```python
from build123d import *

# Parameters (mm, degrees)
SKETCH1_R           = 30
BOSS_EXTRUDE1_DEPTH = 2
SKETCH2_R           = 3.5
SKETCH2_R_2         = 2.5
BOSS_EXTRUDE2_DEPTH = 10
FILLET1_R           = 1
FILLET2_R           = 1


with BuildPart() as part:
    # Sketch1 → Boss-Extrude1 (new body)
    with BuildSketch(Plane(origin=(0, 0, 0), x_dir=(1, 0, 0), z_dir=(0, 1, 0))):
        with Locations(Location((0, 0, 0), (0, 0, 270))):
            Circle(SKETCH1_R)
    extrude(amount=BOSS_EXTRUDE1_DEPTH)

    # Sketch2 → Boss-Extrude2 (add)
    with BuildSketch(Plane.XZ):
        with Locations(Location((0, 0, 0), (0, 0, 90))):
            Circle(SKETCH2_R)
        with Locations(Location((0, 0, 0), (0, 0, 270))):
            Circle(SKETCH2_R_2, mode=Mode.SUBTRACT)
    extrude(amount=BOSS_EXTRUDE2_DEPTH)

    # Fillet1
    fillet1_edges = [part.edges().sort_by_distance(p)[0] for p in [
        (0, 0, -3.5),
    ]]
    fillet(fillet1_edges, radius=FILLET1_R)

    # Fillet2
    fillet2_edges = [part.edges().sort_by_distance(p)[0] for p in [
        (0, 0, 2.5),
    ]]
    fillet(fillet2_edges, radius=FILLET2_R)


solid = part.part
```
Geometry: final body of the model. Coordinates: model frame, mm. A direction names the side the tool comes from. Give positions to 0.01 mm unless a question says otherwise; leave off trailing zeros. Loops run counter-clockwise (first coordinate to the right, second up) from the corner with the lowest first, then second, coordinate; pieces in that order, holes last. Notation, with made-up numbers: (-12, -24.5) -> (20, -24.5) arc R30 ccw to (20, 2.5) -> close; hole circle Ø5 at (64, 51). An arc over 180 degrees is marked (long way). Return JSON: item names as keys, results as strings.
Item 1: Section A-A, the plane x = 0. Output: boundary loops of the cut face in (y, z).
Filled in:
{"outline": "(-10, -3.5) -> (-1, -3.5) arc R1 cw to (0, -4.5) -> (0, -30) -> (2, -30) -> (2, 30) -> (0, 30) -> (0, 4.5) arc R1 cw to (-1, 3.5) -> (-10, 3.5) -> (-10, 2.5) -> (-1, 2.5) arc R1 cw to (0, 1.5) -> (0, -1.5) arc R1 cw to (-1, -2.5) -> (-10, -2.5) -> close"}
Item 2: Pin query (flat end, axial travel): P1, Ø2, axis at x = 21, y = 0, coming from the +Z side; P2, Ø1.5, axis at y = -1, z = -7, coming from the -X side; P3, Ø8, axis at x = 0, z = 0, coming from the -Y side; P4, Ø3, axis at x = 1, z = 5.5, coming from the -Y side. Return the tip coordinate at first contact, or that it passes through.
Filled in:
{"P1": "z = 22.36", "P2": "through", "P3": "y = -10", "P4": "y = -0.09"}
Item 3: Section C-C, the plane y = -7.5. Output: boundary loops of the cut face in (x, z).
Filled in:
{"outline": "circle Ø7 at (0, 0); hole circle Ø5 at (0, 0)"}
Item 4: Section D-D, the plane x = -18. Output: boundary loops of the cut face in (y, z).
Filled in:
{"outline": "(0, -24) -> (2, -24) -> (2, 24) -> (0, 24) -> close"}
Item 5: Line query: line 1 (X direction, y = -6.5, z = 0); line 2 (Y direction, x = -8.5, z = 25); line 3 (X direction, y = -2.25, z = -2). Output: solid intervals per line, ascending.
Filled in:
{"line 1": "-3.5 to -2.5, 2.5 to 3.5", "line 2": "0 to 2", "line 3": "-2.87 to -1.5, 1.5 to 2.87"}
Item 6: Access query for faces 1 (the flat face through (0, 2, 0)), 2 (the cylindrical face through (3.417, -5.437, -0.759)). Directions: +Z, -Z, +X, -X, +Y, -Y. A direction counts if a zero-diameter tool reaches every point of the face in a straight line with its end or side. Return the directions, or none.
Filled in:
{"face 1": "+Z, -Z, +X, -X, +Y", "face 2": "-Y"}
Item 7: Section B-B, the plane z = 0. Output: boundary loops of the cut face in (x, y), plus the area to 3 significant figures.
Filled in:
{"outline": "(-30, 0) -> (-4.5, 0) arc R1 cw to (-3.5, -1) -> (-3.5, -10) -> (-2.5, -10) -> (-2.5, -1) arc R1 cw to (-1.5, 0) -> (1.5, 0) arc R1 cw to (2.5, -1) -> (2.5, -10) -> (3.5, -10) -> (3.5, -1) arc R1 cw to (4.5, 0) -> (30, 0) -> (30, 2) -> (-30, 2) -> close", "area": "141 mm^2"}
Item 8: Mould query, pull axis X, two halves, no side actions, for faces 3 (the flat face through (0, 0, 6)), 4 (the flat face through (0, 0, 0)), 5 (the cylindrical face through (1.32, 0.99, -29.97)), 6 (the cylindrical face through (-2.44, -5.44, 0.54)). Classes: released by +X, released by -X, zero draft, split by the parting line, or undercut.
Filled in:
{"face 3": "zero draft", "face 4": "undercut", "face 5": "split by the parting line", "face 6": "undercut"}
